from build123d import *

# Parameters (mm, degrees)
CROQUIS1_R              = 5
BASE_DEPTH              = 30
CROQUIS4_R              = 7.5
CORTAR_EXTRUIR3_DEPTH   = 64.725975865
CROQUIS7_W              = 10
CROQUIS7_H              = 28.5
CORTAR_EXTRUIR6_DEPTH   = 64.725975865
CROQUIS8_W              = 44
CROQUIS8_H              = 8
CORTAR_EXTRUIR7_DEPTH   = 52.078371156
REDONDEO3_R             = 5
CROQUIS10_R             = 7.5
CROQUIS10_R_2           = 6.5
SALIENTE_EXTRUIR2_DEPTH = 10


with BuildPart() as part:
    # Croquis1 → Base (new body)
    with BuildSketch(Plane.XY):
        Polygon((-10, 35), (-22, 35), (-22, -35), (22, -35), (22, 35), (10, 35), (10, 15), (-10, 15), align=None)
        with Locations((0, -20.5)):
            Circle(CROQUIS1_R, mode=Mode.SUBTRACT)
    extrude(amount=BASE_DEPTH)

    # Croquis4 → Cortar-Extruir3 (cut, through all)
    with BuildSketch(Plane(origin=(22, 0, 0), x_dir=(0, 0, -1), z_dir=(1, 0, 0))):
        with Locations(Location((-15, 5, 0), (0, 0, 90))):
            Circle(CROQUIS4_R)
    extrude(amount=-CORTAR_EXTRUIR3_DEPTH, mode=Mode.SUBTRACT)

    # Croquis7 → Cortar-Extruir6 (cut, through all)
    with BuildSketch(Plane(origin=(22, 0, 0), x_dir=(0, 0, -1), z_dir=(1, 0, 0))):
        with Locations((-15, -20.75)):
            Rectangle(CROQUIS7_W, CROQUIS7_H)
    extrude(amount=-CORTAR_EXTRUIR6_DEPTH, mode=Mode.SUBTRACT)

    # Croquis8 → Cortar-Extruir7 (cut, through all)
    with BuildSketch(Plane.XY.offset(30)):
        with Locations((0, -31)):
            Rectangle(CROQUIS8_W, CROQUIS8_H)
    extrude(amount=-CORTAR_EXTRUIR7_DEPTH, mode=Mode.SUBTRACT)

    # Redondeo3
    redondeo3_edges = [part.edges().sort_by_distance(p)[0] for p in [
        (-22, -27, 25),
        (-22, -27, 5),
        (22, -27, 25),
        (22, -27, 5),
    ]]
    fillet(redondeo3_edges, radius=REDONDEO3_R)

    # Croquis10 → Saliente-Extruir2 (add)
    with BuildSketch(Plane(origin=(22, 0, 0), x_dir=(0, 0, -1), z_dir=(1, 0, 0))):
        with Locations(Location((-15, 5, 0), (0, 0, 90))):
            Circle(CROQUIS10_R)
        with Locations(Location((-15, 5, 0), (0, 0, 90))):
            Circle(CROQUIS10_R_2, mode=Mode.SUBTRACT)
    extrude(amount=-SALIENTE_EXTRUIR2_DEPTH)


solid = part.part
Input: part model. Units: mm. Frame: model coordinates. A direction names the side the tool comes from. Round coordinates to 2 decimals unless told otherwise and drop trailing zeros. Loops run counter-clockwise (first coordinate to the right, second up) from the corner with the lowest first, then second, coordinate; pieces in that order, holes last. Notation, with made-up numbers: (46.5, 36) -> (83.5, 36) arc R15 ccw to (83.5, 53) -> close; hole circle Ø5 at (26, 30). An arc over 180 degrees is marked (long way). Answer as a JSON object with one key per item and string values. Group by question number.
1) Ray query, L1, parallel to X at y = -20.5, z = 25.5; L2, parallel to Z at x = -19, y = -20; L3, parallel to X at y = 20, z = 8.5. Return the intervals inside material, ascending.
2) Draft query along Z for faces 5 (the flat face through (0, -15, 20)), 6 (the flat face through (22, 12, 15)), 7 (the flat face through (0, 4, 30)). Return one class per face: +Z half, -Z half, draft (parallel to the pull), parting line (faces both ways), or undercut.
3) Section query A-A on x = 0. Output: boundary loops of the cut face in (y, z), plus the area to 3 significant figures.
4) Section query C-C on y = -20.5. Output: boundary loops of the cut face in (x, z), plus the area to 3 significant figures.
5) Section query B-B on z = 15. Output: boundary loops of the cut face in (x, y), plus the area to 3 significant figures.
6) Pin query (flat end, axial travel): pin 1 (8 mm diameter, centred on x = -9, z = 14.5, fed in from -Y); pin 2 (1.5 mm diameter, centred on x = -4, z = 26, fed in from +Y); pin 3 (9 mm diameter, centred on x = 0, y = -20.5, fed in from -Z). Return the tip coordinate at first contact, or that it passes through.
7) Reachability of faces 1 (the flat face through (-10, 25, 15)), 2 (the cylindrical face through (-4.762, 9.032, 21.324)), 3 (the flat face through (0, -15, 10)), 4 (the flat face through (-22, 13, 15)) from +Z, -Z, +X, -X, +Y, -Y: full face, straight path, thin tool, end or side. Return the list, or none.
8) Section query D-D on y = -8. Output: boundary loops of the cut face in (x, z).
Reply:
{
 "1": {"L1": "x = -22 to -5, 5 to 22", "L2": "z = 0 to 10, 20 to 30", "L3": "x = -22 to -10, 10 to 22"},
 "2": {"face 5": "undercut", "face 6": "draft", "face 7": "+Z half"},
 "3": {"outline": "(-27, 0) -> (-25.5, 0) -> (-25.5, 10) -> (-27, 10) -> close; (-27, 20) -> (-25.5, 20) -> (-25.5, 30) -> (-27, 30) -> close; (-15.5, 0) -> (15, 0) -> (15, 30) -> (-15.5, 30) -> (-15.5, 20) -> (-6.5, 20) -> (-6.5, 10) -> (-15.5, 10) -> close; hole circle Ø15 at (5, 15)", "area": "678 mm2"},
 "4": {"outline": "(-22, 0) -> (-5, 0) -> (-5, 10) -> (-22, 10) -> close; (-22, 20) -> (-5, 20) -> (-5, 30) -> (-22, 30) -> close; (5, 0) -> (22, 0) -> (22, 10) -> (5, 10) -> close; (5, 20) -> (22, 20) -> (22, 30) -> (5, 30) -> close", "area": "680 mm2"},
 "5": {"outline": "(-22, -6.5) -> (22, -6.5) -> (22, -1.5) -> (12, -1.5) -> (12, -2.5) -> (-22, -2.5) -> close; (-22, 12.5) -> (12, 12.5) -> (12, 11.5) -> (22, 11.5) -> (22, 35) -> (10, 35) -> (10, 15) -> (-10, 15) -> (-10, 35) -> (-22, 35) -> close", "area": "786 mm2"},
 "6": {"pin 1": "stops at y = -6.5", "pin 2": "stops at y = 15", "pin 3": "passes through"},
 "7": {"face 1": "+Z, -Z, +Y", "face 2": "-X", "face 3": "+X, -X, -Y", "face 4": "+Z, -Z, -X, +Y, -Y"},
 "8": {"outline": "(-22, 0) -> (22, 0) -> (22, 10) -> (-22, 10) -> close; (-22, 20) -> (22, 20) -> (22, 30) -> (-22, 30) -> close"}
}
